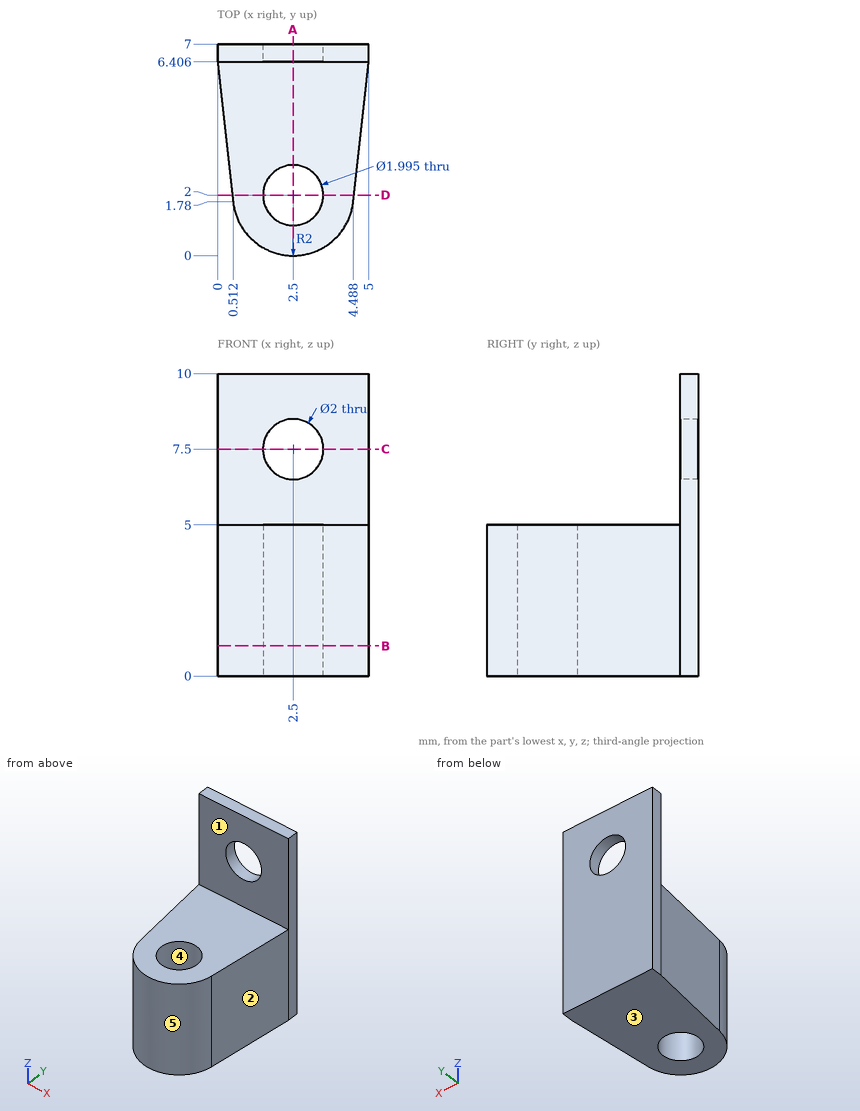
Part print with two shaded views. Sizes in mm from the minimum x, y, z corner. A direction names the side the tool comes from. Give positions to 0.01 mm unless a question says otherwise; leave off trailing zeros. Order: outer loops, then holes, each group sorted by start corner. A loop starts at its lowest first (then second) coordinate and runs counter-clockwise, first axis right, second up.
(1) Saw through at B-B, the plane z = 1. Give the cut face in (x, y) (1 decimal).
(2) Drill centre lines: L1, parallel to Z at x = 1.95, y = 5.25; L2, parallel to Y at x = 4.3, z = 9.75; L3, parallel to Y at x = 2.15, z = 4.5 (1 decimal). Where is each one in solid material? Low to high.
(3) Saw through at A-A, the plane x = 2.5. Give the cut face in (y, z), then the cut area to 3 significant figures.
(4) Flat gauge pins, fed straight in: pin 1 (1.5 mm diameter, centred on x = 1.5, y = 2, fed in from -Z); pin 2 (4 mm diameter, centred on y = 3.5, z = 6.5, fed in from +X) (1 decimal); pin 3 (2.5 mm diameter, centred on x = 3, y = 4.5, fed in from +Z). Where does each tip first touch, or does it go through?
(5) Saw through at D-D, the plane y = 2. Give the cut face in (x, z).
(6) Mould opens along X. For the marked faces 3, 4 and 5 say: released by +X, released by -X, zero draft, split by the parting line, or undercut.
(7) Saw through at C-C, the plane z = 7.5. Give the cut face in (x, y).
(8) Tool access for the marked faces 1 and 2: list every direction of +Z, -Z, +X, -X, +Y, -Y with a clear straight run to the whole face (end or side of a thin tool).
Results found:
1. outline: (0, 6.4) - (0.5, 1.8) arc R2 ccw to (4.5, 1.8) - (5, 6.4) - (5, 7) - (0, 7) - close; hole circle Ø2 at (2.5, 2)
2. L1: z = 0 to 5
2. L2: y = 6.41 to 7
2. L3: y = 0 to 1.1, 2.9 to 7
3. outline: (0, 0) - (1, 0) - (1, 5) - (0, 5) - close; (3, 0) - (7, 0) - (7, 6.5) - (6.41, 6.5) - (6.41, 5) - (3, 5) - close; (6.41, 8.5) - (7, 8.5) - (7, 10) - (6.41, 10) - close
3. area: 26.8 mm2
4. pin 1: stops at z = 0
4. pin 2: stops at x = 4.8
4. pin 3: stops at z = 5
5. outline: (0.49, 0) - (1.5, 0) - (1.5, 5) - (0.49, 5) - close; (3.5, 0) - (4.51, 0) - (4.51, 5) - (3.5, 5) - close
6. face 3: zero draft
6. face 4: undercut
6. face 5: split by the parting line
7. outline: (0, 6.41) - (1.5, 6.41) - (1.5, 7) - (0, 7) - close; (3.5, 6.41) - (5, 6.41) - (5, 7) - (3.5, 7) - close
8. face 1: +Z, +X, -X, -Y
8. face 2: +Z, -Z, +X, -Y
